from build123d import *

# Parameters (mm, degrees)
F0_W     = 120
F0_H     = 120
F1_DEPTH = 10
F2_W     = 112
F2_H     = 10
F3_DEPTH = 6
F5_D     = 5


with BuildPart() as f1:
    # F0 (on Top) → F1 (new body)
    with BuildSketch(Plane.XY):
        with Locations((60, 60)):
            Rectangle(F0_W, F0_H)
    extrude(amount=F1_DEPTH)

    # F2 (on face) → F3 (cut)
    with BuildSketch(Plane(origin=(0, 0, 0), x_dir=(1, 0, 0), z_dir=(0, 0, -1))):
        with Locations((60, -105)):
            Rectangle(F2_W, F2_H)
        with Locations((60, -35)):
            Rectangle(F2_W, F2_H)
    extrude(amount=-F3_DEPTH, mode=Mode.SUBTRACT)

    # F5 (through all)
    with Locations(Plane.XY.offset(10)):
        with Locations((45, 70), (75, 70)):
            Hole(F5_D / 2)


solid = f1.part
Check sheet for the modelled part. Datum: model origin and axes. Units: mm. A direction names the side the tool comes from. Give positions to 0.01 mm unless a question says otherwise; leave off trailing zeros. Write each loop counter-clockwise with the first axis right and the second up, starting at its lowest first coordinate (ties: lowest second). Pieces come first, ordered by that corner, then holes. Notation, with made-up numbers: (70.25, 43.5) -> (108.25, 43.5) arc R27 cw to (108.25, 63.5) -> close; hole circle Ø3 at (7.25, -18.5). An arc over 180 degrees is marked (long way). Write item = value, one per line.
Item 1: Tool access check on faces 4 (the flat face through (0, 59, 5)), 5 (the flat face through (59, 35, 6)). Record the directions out of +Z, -Z, +X, -X, +Y, -Y that give a thin tool (end or side, any length) a straight path to the whole face; none if there is none.
Output:
face_4 = +Z, -Z, -X, +Y, -Y
face_5 = -Z
Item 2: Sectioned sample at A-A on x = 45. Record the boundary of the cut face in (y, z).
Output:
outline = (0, 0) -> (30, 0) -> (30, 6) -> (40, 6) -> (40, 0) -> (67.5, 0) -> (67.5, 10) -> (0, 10) -> close; (72.5, 0) -> (100, 0) -> (100, 6) -> (110, 6) -> (110, 0) -> (120, 0) -> (120, 10) -> (72.5, 10) -> close
Item 3: Sectioned sample at B-B on z = 3.5. Record the boundary of the cut face in (x, y), and give its area (3 significant figures).
Output:
outline = (0, 0) -> (120, 0) -> (120, 120) -> (0, 120) -> close; hole (4, 30) -> (116, 30) -> (116, 40) -> (4, 40) -> close; hole (4, 100) -> (116, 100) -> (116, 110) -> (4, 110) -> close; hole circle Ø5 at (45, 70); hole circle Ø5 at (75, 70)
area = 12,100 mm^2
Item 4: Gauge pin test, flat end, axial feed: pin 1 (4 mm diameter, centred on x = 16.5, y = 104.5, fed in from -Z). Record the tip position at first contact, or that the pin passes through.
Output:
pin_1 = 6
Item 5: Sectioned sample at D-D on y = 34. Record the boundary of the cut face in (x, z).
Output:
outline = (0, 0) -> (4, 0) -> (4, 6) -> (116, 6) -> (116, 0) -> (120, 0) -> (120, 10) -> (0, 10) -> close
Item 6: Sectioned sample at C-C on y = 70. Record the boundary of the cut face in (x, z).
Output:
outline = (0, 0) -> (42.5, 0) -> (42.5, 10) -> (0, 10) -> close; (47.5, 0) -> (72.5, 0) -> (72.5, 10) -> (47.5, 10) -> close; (77.5, 0) -> (120, 0) -> (120, 10) -> (77.5, 10) -> close
Item 7: Scan lines: probe 1 along Y at (x, z) = (35, 1); probe 2 along Y at (x, z) = (75, 4.75); probe 3 along X at (y, z) = (106, 2). Record each from-to range of solid material in increasing order. Write a range as from..to.
Output:
probe_1 = 0..30, 40..100, 110..120
probe_2 = 0..30, 40..67.5, 72.5..100, 110..120
probe_3 = 0..4, 116..120
Item 8: Release check for a two-part mould opening along Y. For faces 1 (the flat face through (59, 110, 3)), 2 (the flat face through (59, 120, 5)), 3 (the flat face through (59, 61, 10)) record: +Y half, -Y half, draft (parallel to the pull), parting line (faces both ways), or undercut.
Output:
face_1 = undercut
face_2 = +Y half
face_3 = draft
